```python
from build123d import *

# Parameters (mm, degrees)
SKETCH1_R           = 3.5
BOSS_EXTRUDE1_DEPTH = 30


with BuildPart() as part:
    # Sketch1 → Boss-Extrude1 (new body)
    with BuildSketch(Plane.XY):
        with BuildLine():
            Line((3.541917671, 25), (5.463208389, 24.444444444))
            ThreePointArc((5.463208389, 24.444444444), (5.24739546, 23.685354625), (5.038398555, 22.924359969))
            ThreePointArc((5.038398555, 22.924359969), (10.794070727, 16.953488372), (3.098606761, 13.861740626))
            ThreePointArc((3.098606761, 13.861740626), (2, 0), (3.098606761, -13.861740626))
            ThreePointArc((3.098606761, -13.861740626), (10.794070727, -16.953488372), (5.038398555, -22.924359969))
            ThreePointArc((5.038398555, -22.924359969), (5.24739546, -23.685354625), (5.463208389, -24.444444444))
            Line((5.463208389, -24.444444444), (3.541917671, -25))
            ThreePointArc((3.541917671, -25), (3.099888289, -23.417313778), (2.686828675, -21.826820958))
            ThreePointArc((2.686828675, -21.826820958), (1.01556094, -19.046511628), (1.402328405, -15.825693915))
            ThreePointArc((1.402328405, -15.825693915), (0, 0), (1.402328405, 15.825693915))
            ThreePointArc((1.402328405, 15.825693915), (1.01556094, 19.046511628), (2.686828675, 21.826820958))
            ThreePointArc((2.686828675, 21.826820958), (3.099888289, 23.417313778), (3.541917671, 25))
        make_face()
        with Locations((5.904815833, 18)):
            Circle(SKETCH1_R, mode=Mode.SUBTRACT)
        with Locations((5.904815833, -18)):
            Circle(SKETCH1_R, mode=Mode.SUBTRACT)
    extrude(amount=BOSS_EXTRUDE1_DEPTH)


solid = part.part
```
Geometry check sheet. Reference: the model listing, model coordinates, mm. Coordinates: 2 decimals unless noted, no trailing zeros. Order: outer loops, then holes, each group sorted by start corner. A loop starts at its lowest first (then second) coordinate and runs counter-clockwise, first axis right, second up. Notation, with made-up numbers: M 18.5,30.25 L 55.5,30.25 A10 cw 55.5,34.25 Z; hole C 82,-21.5 d5. An arc over 180 degrees is marked long. Answer as a JSON object with one key per item and string values.
Q1. Cross-section at A-A on y = -18. Record the cut outline in (x, z), and give its area (3 significant figures).
Results are:
{"outline": "M 0.9,0 L 2.4,0 L 2.4,30 L 0.9,30 Z; M 9.4,0 L 10.9,0 L 10.9,30 L 9.4,30 Z", "area": "90.0 mm²"}
Q2. Cross-section at B-B on z = 15. Record the cut outline in (x, y).
Results are:
{"outline": "M 1.4,-15.83 A5 ccw 2.69,-21.83 A90 ccw 3.54,-25 L 5.46,-24.44 A88 cw 5.04,-22.92 A5 ccw long 3.1,-13.86 A88 cw 3.1,13.86 A5 ccw long 5.04,22.92 A88 cw 5.46,24.44 L 3.54,25 A90 ccw 2.69,21.83 A5 ccw 1.4,15.83 A90 ccw Z; hole C 5.9,-18 d7; hole C 5.9,18 d7"}
Q3. Release check for a two-part mould opening along Y. For faces 1 (the flat face through (1.8, -1.7, 0)), 2 (the cylindrical face through (1.006, 19.001, 14.79)), 3 (the cylindrical face through (3.106, -23.44, 14.79)) record: released by +Y, released by -Y, zero draft, split by the parting line, or undercut.
Results are:
{"face 1": "zero draft", "face 2": "undercut", "face 3": "released by -Y"}
Q4. Scan lines: line 1 (Y direction, x = 8, z = 26.5); line 2 (Y direction, x = 8.75, z = 9.25); line 3 (X direction, y = -16.5, z = 27.25). Record each from-to range of solid material in increasing order.
Results are:
{"line 1": "y = -22.54 to -20.8, -15.2 to -13.46, 13.46 to 15.2, 20.8 to 22.54", "line 2": "y = -22.11 to -20.04, -15.96 to -13.89, 13.89 to 15.96, 20.04 to 22.11", "line 3": "x = 1.14 to 2.74, 9.07 to 10.67"}
Q5. Depth check by flat-ended pin: pin 1 Ø12 at (y, z) = (-6.5, 22) entering from -X; pin 2 Ø3 at (x, z) = (6, 17) entering from +Y; pin 3 Ø5 at (x, z) = (7.5, 6) entering from -Y; pin 4 Ø3 at (x, y) = (8, -12) entering from -Z. Enter the tip coordinate at first touch or a pass-through.
Results are:
{"pin 1": "stops at x = 0", "pin 2": "stops at y = 24.72", "pin 3": "stops at y = -24.58", "pin 4": "stops at z = 0"}
Q6. Cross-section at C-C on x = 6. Record the cut outline in (y, z), and give its area (3 significant figures).
Results are:
{"outline": "M -23,0 L -21.5,0 L -21.5,30 L -23,30 Z; M -14.5,0 L -13,0 L -13,30 L -14.5,30 Z; M 13,0 L 14.5,0 L 14.5,30 L 13,30 Z; M 21.5,0 L 23,0 L 23,30 L 21.5,30 Z", "area": "180 mm²"}
Q7. Cross-section at D-D on y = -9.5. Record the cut outline in (x, z).
Results are:
{"outline": "M 0.5,0 L 2.51,0 L 2.51,30 L 0.5,30 Z"}
